Verification items for the finished model (mm, model axes). A direction names the side the tool comes from. Round coordinates to 2 decimals unless told otherwise and drop trailing zeros. Write each loop counter-clockwise with the first axis right and the second up, starting at its lowest first coordinate (ties: lowest second). Pieces come first, ordered by that corner, then holes. Notation, with made-up numbers: (2, 15.25) -> (31, 15.25) arc R10 cw to (31, 20.25) -> close; hole circle Ø10 at (33.5, -17.5). An arc over 180 degrees is marked (long way). Answer as a JSON object with one key per item and string values. Group by question number.
(1) Scan lines: L1, parallel to Z at x = 0, y = -2.75; L2, parallel to Z at x = -10, y = 8.5; L3, parallel to Y at x = -0.5, z = -33. Record each from-to range of solid material in increasing order. Write a range as from..to.
(2) Sectioned sample at B-B on y = -14. Record the cut outline in (x, z), and give its area (3 significant figures).
(3) Set-up check for faces 1 (the face through (-13.887, -10.648, -312.325)), 2 (the face through (-1.08, 0.11, -4.88)), 3 (the face through (4, -7.5, -4)), 4 (the face through (-7.493, 0.33, -161.24)): record each of +Z, -Z, +X, -X, +Y, -Y from which the full face is reachable in a straight line by a thin tool's end or side.
(4) Gauge pin test, flat ends, axial feed: pin 1 Ø6 at (x, z) = (9, -267) entering from -Y; pin 2 Ø12 at (y, z) = (-7, -76) entering from -X; pin 3 Ø16 at (x, z) = (0, 0) entering from +Y. Record the tip position at first contact, or that the pin passes through.
(5) Sectioned sample at A-A on z = 0. Record the cut outline in (x, y), and give its area (3 significant figures).
(6) Sectioned sample at C-C on z = -191. Record the cut outline in (x, y).
(7) Draft check along Z on faces 5 (the face through (0, -8, -300)), 6 (the face through (0, 0, -325)), 7 (the face through (4, 7.5, -4)). Enter one of: released by +Z, released by -Z, zero draft, split by the parting line, or undercut.
```python
from build123d import *

# Parameters (mm, degrees)
F0_R     = 20
F0_R_2   = 5
F1_DEPTH = 7.5
F3_R     = 7.5
F5_R     = 17.5
F6_DEPTH = 25


with BuildPart() as f1:
    # F0 (on Front) → F1 (new body, symmetric)
    with BuildSketch(Plane.XZ):
        Circle(F0_R)
        Circle(F0_R_2, mode=Mode.SUBTRACT)
    extrude(amount=F1_DEPTH, both=True)

    # F3 (on offset) → F4 (join, up to the next surface of F1)
    with BuildSketch(Plane.XY.offset(-300)):
        Circle(F3_R)
    extrude(until=Until.NEXT)

    # F5 (on offset) → F6 (join)
    with BuildSketch(Plane.XY.offset(-300)):
        Circle(F5_R)
    extrude(amount=-F6_DEPTH)


solid = f1.part
```
Computed values:
{
 "1": {"L1": "-325..-5, 5..20", "L2": "-325..-300", "L3": "-7.48..7.48"},
 "2": {"outline": "(-10.5, -325) -> (10.5, -325) -> (10.5, -300) -> (-10.5, -300) -> close", "area": "525 mm2"},
 "3": {"face 1": "-Z", "face 2": "+Y, -Y", "face 3": "+Z, +X, -X, -Y", "face 4": "none"},
 "4": {"pin 1": "y = -4.5", "pin 2": "x = -7.43", "pin 3": "y = 7.5"},
 "5": {"outline": "(-20, -7.5) -> (-5, -7.5) -> (-5, 7.5) -> (-20, 7.5) -> close; (5, -7.5) -> (20, -7.5) -> (20, 7.5) -> (5, 7.5) -> close", "area": "450 mm2"},
 "6": {"outline": "circle Ø15 at (0, 0)"},
 "7": {"face 5": "undercut", "face 6": "released by -Z", "face 7": "zero draft"}
}
